Geometry: final body of the model. Coordinates: model frame, mm. Face numbers are marked on the shaded views. A direction names the side the tool comes from. Give positions to 0.01 mm unless a question says otherwise; leave off trailing zeros. Write each loop counter-clockwise with the first axis right and the second up, starting at its lowest first coordinate (ties: lowest second). Pieces come first, ordered by that corner, then holes.
from build123d import *

# Parameters (mm, degrees)
F2_R     = 17.6784
F3_DEPTH = 3.1242
F5_DEPTH = 6.8961
F7_DEPTH = 7.62


with BuildPart() as f1:
    # F0 (on Front) → F1 (revolve)
    with BuildSketch(Plane.XZ):
        Polygon((0, 21.1963), (0, 0), (12.2428, 0), (12.2428, 3.5433), (10.48385, 3.5433), (10.48385, 7.4803), (12.2428, 7.4803), (12.2428, 10.0203), (4.2291, 10.0203), (4.2291, 16.6497), (2.5654, 16.6497), (2.5654, 19.9263), (4.2291, 19.9263), (4.2291, 21.1963), align=None)
    revolve(axis=Axis((0, 0, 10.59815), (0, 0, 1)))

    # F2 (on face) → F3 (join)
    with BuildSketch(Plane(origin=(0, 0, 0), x_dir=(1, 0, 0), z_dir=(0, 0, -1))):
        Circle(F2_R)
    extrude(amount=F3_DEPTH)

    # F4 (on face) → F5 (join)
    with BuildSketch(Plane(origin=(0, 0, -3.1242), x_dir=(1, 0, 0), z_dir=(0, 0, -1))):
        with BuildLine():
            Line((-13.0175, 11.961209), (-13.0175, -11.961209))
            ThreePointArc((-13.0175, -11.961209), (0, -17.6784), (13.0175, -11.961209))
            Line((13.0175, -11.961209), (13.0175, 11.961209))
            ThreePointArc((13.0175, 11.961209), (0, 17.6784), (-13.0175, 11.961209))
        make_face()
    extrude(amount=F5_DEPTH)

    # F6 (on face) → F7 (join)
    with BuildSketch(Plane(origin=(0, 0, -10.0203), x_dir=(1, 0, 0), z_dir=(0, 0, -1))):
        with BuildLine():
            ThreePointArc((-6.477, -16.449143), (0, -17.6784), (6.477, -16.449143))
            Line((6.477, -16.449143), (6.477, 16.449143))
            ThreePointArc((6.477, 16.449143), (0, 17.6784), (-6.477, 16.449143))
            Line((-6.477, 16.449143), (-6.477, -16.449143))
        make_face()
        with BuildLine():
            Line((-6.477, -27.94), (6.477, -27.94))
            Line((6.477, -27.94), (6.477, -16.449143))
            ThreePointArc((6.477, -16.449143), (0, -17.6784), (-6.477, -16.449143))
            Line((-6.477, -16.449143), (-6.477, -27.94))
        make_face()
    extrude(amount=F7_DEPTH)


solid = f1.part
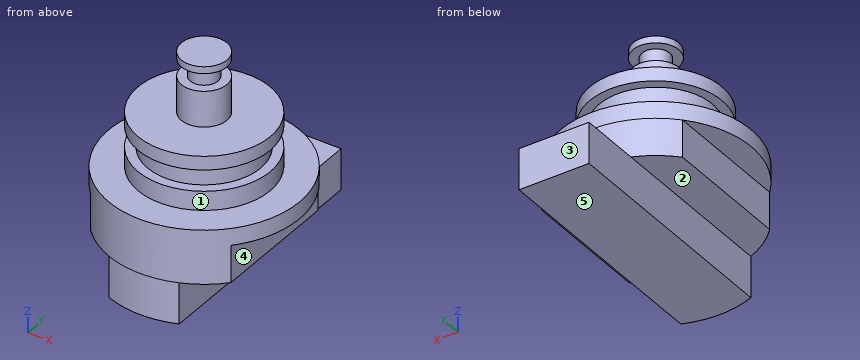
Q1. Section D-D on y = 15. Output: boundary loops of the cut face in (x, z), plus the area to 3 significant figures.
Filled sheet:
outline: (-9.36, -10.02) - (-6.48, -10.02) - (-6.48, -17.64) - (6.48, -17.64) - (6.48, -10.02) - (9.36, -10.02) - (9.36, 0) - (-9.36, 0) - close
area: 286 mm2
Q2. Access query for the marked faces 1, 2, 3, 4 and 5. Directions: +Z, -Z, +X, -X, +Y, -Y. A direction counts if a zero-diameter tool reaches every point of the face in a straight line with its end or side. Return the directions, or none.
Filled sheet:
face 1: +Z
face 2: -Z, -X, +Y, -Y
face 3: +Z, -Z, +X, -X, +Y
face 4: -Z, +X, +Y, -Y
face 5: -Z, +X, -X, +Y, -Y
Q3. Section B-B on y = 5. Output: boundary loops of the cut face in (x, z), plus the area to 3 significant figures.
Filled sheet:
outline: (-16.96, -3.12) - (-13.02, -3.12) - (-13.02, -10.02) - (-6.48, -10.02) - (-6.48, -17.64) - (6.48, -17.64) - (6.48, -10.02) - (13.02, -10.02) - (13.02, -3.12) - (16.96, -3.12) - (16.96, 0) - (11.18, 0) - (11.18, 3.54) - (9.21, 3.54) - (9.21, 7.48) - (11.18, 7.48) - (11.18, 10.02) - (-11.18, 10.02) - (-11.18, 7.48) - (-9.21, 7.48) - (-9.21, 3.54) - (-11.18, 3.54) - (-11.18, 0) - (-16.96, 0) - close
area: 593 mm2
Q4. Section C-C on z = 13. Output: boundary loops of the cut face in (x, y), plus the area to 3 significant figures.
Filled sheet:
outline: circle Ø8.46 at (0, 0)
area: 56.2 mm2
Q5. Ray query, line 1 along Z through (x, y) = (3, -2); line 2 along Z through (x, y) = (10.5, 1); line 3 along X through (y, z) = (-0.5, -3). Return the intervals inside material, ascending.
Filled sheet:
line 1: z = -17.64 to 16.65, 19.93 to 21.2
line 2: z = -10.02 to 3.54, 7.48 to 10.02
line 3: x = -17.67 to 17.67
Q6. Pin query (flat end, axial travel): P1, Ø3.5, axis at x = 9, y = -3.5, coming from the -Z side; P2, Ø12, axis at y = 14, z = -7.5, coming from the +X side; P3, Ø7.5, axis at y = -5, z = -5, coming from the -X side; P4, Ø12, axis at x = 7, y = 3.5, coming from the -Z side. Return the tip coordinate at first contact, or that it passes through.
Filled sheet:
P1: stops at z = -10.02
P2: stops at x = 14.65
P3: stops at x = -17.59
P4: stops at z = -17.64
